Could you check a few things on this drawing? It's one solid part, dimensions in mm from its lowest x, y, z. Give positions to 0.01 mm unless a question says otherwise; leave off trailing zeros. Loops run counter-clockwise (first coordinate to the right, second up) from the corner with the lowest first, then second, coordinate; pieces in that order, holes last. Notation, with made-up numbers: M -35,62.5 L -20,62.5 A12 cw -20,67.5 Z; hole C -5.75,60 d3. An arc over 180 degrees is marked long. One line per item, written item: value. Start each with the question number.
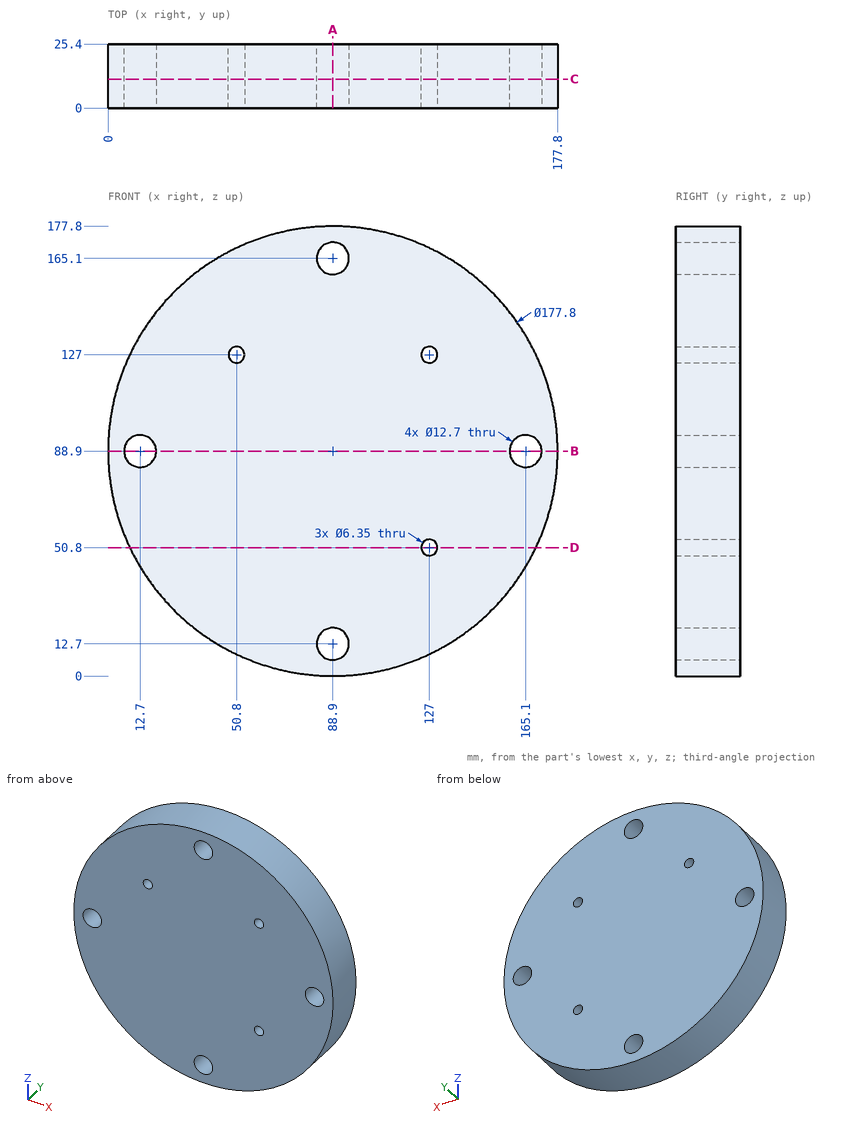
Q1. If we section it at A-A, the plane x = 88.9: Write out the boundary of the cut face in (y, z), plus the area to 3 significant figures.
Q2. If we section it at B-B, the plane z = 88.9: Write out the boundary of the cut face in (x, y), plus the area to 3 significant figures.
Q3. For P1, Ø7.5, axis at x = 88.9, z = 165.1, coming from the -Y side; P2, Ø3, axis at x = 66.5, y = 7.5, coming from the +Z side; P3, Ø2, axis at x = 125, y = 10, coming from the -Z side; P4, Ø1, axis at y = 22.5, z = 124.5, coming from the -X side, each with a flat end and sliding along its axis, tell me the tip position at first contact or that it passes through.
Q4. If we section it at C-C, the plane y = 11.5: Write out the boundary of the cut face in (x, z) (3 decimals), plus the area to 3 significant figures.
Q5. I need wall thicknesses on line 1 along X through (y, z) = (4, 92); line 2 along X through (y, z) = (5.5, 83.5); line 3 along Z through (x, y) = (127, 14.75) (3 decimals). Which ranges of each line are inside material? Lowest first, please.
Q6. If we section it at D-D, the plane z = 50.8: Write out the boundary of the cut face in (x, y) (3 decimals), plus the area to 3 significant figures.
Response:
1. outline: M 0,0 L 25.4,0 L 25.4,6.35 L 0,6.35 Z; M 0,19.05 L 25.4,19.05 L 25.4,158.75 L 0,158.75 Z; M 0,171.45 L 25.4,171.45 L 25.4,177.8 L 0,177.8 Z
1. area: 3,870 mm^2
2. outline: M 0,0 L 6.35,0 L 6.35,25.4 L 0,25.4 Z; M 19.05,0 L 158.75,0 L 158.75,25.4 L 19.05,25.4 Z; M 171.45,0 L 177.8,0 L 177.8,25.4 L 171.45,25.4 Z
2. area: 3,870 mm^2
3. P1: through
3. P2: z = 175.31
3. P3: z = 7.22
3. P4: x = 7.22
4. outline: C 88.9,88.9 d177.8; hole C 12.7,88.9 d12.7; hole C 50.8,127 d6.35; hole C 88.9,12.7 d12.7; hole C 88.9,165.1 d12.7; hole C 127,50.8 d6.35; hole C 127,127 d6.35; hole C 165.1,88.9 d12.7
4. area: 24,200 mm^2
5. line 1: 0.05 to 7.16, 18.24 to 159.56, 170.64 to 177.75
5. line 2: 0.16 to 9.36, 16.04 to 161.76, 168.44 to 177.64
5. line 3: 8.578 to 47.625, 53.975 to 123.825, 130.175 to 169.222
6. outline: M 8.578,0 L 123.825,0 L 123.825,25.4 L 8.578,25.4 Z; M 130.175,0 L 169.222,0 L 169.222,25.4 L 130.175,25.4 Z
6. area: 3,920 mm^2
